The model under review builds one solid part; all positions refer to its coordinate system, in mm. A direction names the side the tool comes from. Round coordinates to 2 decimals unless told otherwise and drop trailing zeros. Write each loop counter-clockwise with the first axis right and the second up, starting at its lowest first coordinate (ties: lowest second). Pieces come first, ordered by that corner, then holes. Notation, with made-up numbers: (47, 83) -> (72, 83) arc R31 cw to (72, 120) -> close; hole circle Ø11 at (63.25, 89). An arc over 180 degrees is marked (long way). Answer in a Markdown table with one row per item. Add a question column.
```python
from build123d import *

# Parameters (mm, degrees)
BASE_FLANGE1_DEPTH = 70
CUT_EXTRUDE1_REACH = 78.974
CUT_EXTRUDE2_REACH = 78.348
SKETCH7_R          = 9
CUT_EXTRUDE3_REACH = 75.866
SKETCH8_R          = 3.25
FILLET1_R          = 1


# Sheet-metal steps are written as plain solids
with BuildPart() as part:
    # Sketch1 → Base-Flange1 (new body)
    with BuildSketch(Plane(origin=(0, 0, 0), x_dir=(0, 0, -1), z_dir=(1, 0, 0))):
        with BuildLine():
            Line((-12.5, 20), (-12.5, 3))
            ThreePointArc((-12.5, 3), (-11.621320344, 0.878679656), (-9.5, 0))
            Line((-9.5, 0), (9.5, 0))
            ThreePointArc((9.5, 0), (11.621320344, 0.878679656), (12.5, 3))
            Line((12.5, 3), (12.5, 20))
            Line((12.5, 20), (10.5, 20))
            Line((10.5, 20), (10.5, 3))
            ThreePointArc((10.5, 3), (10.207106781, 2.292893219), (9.5, 2))
            Line((9.5, 2), (-9.5, 2))
            ThreePointArc((-9.5, 2), (-10.207106781, 2.292893219), (-10.5, 3))
            Line((-10.5, 3), (-10.5, 20))
            Line((-10.5, 20), (-12.5, 20))
        make_face()
    extrude(amount=BASE_FLANGE1_DEPTH)

    # Sketch6 → Cut-Extrude1 (cut, up to next)
    with BuildSketch(Plane.XY.offset(12.5), mode=Mode.PRIVATE) as cut_extrude1_sk1:
        Polygon((35, 8.952994616), (45, 14.726497308), (45, 26.273502692), (35, 32.047005384), (25, 26.273502692), (25, 14.726497308), align=None)
    cut_extrude1_tool1 = extrude(cut_extrude1_sk1.sketch, amount=-CUT_EXTRUDE1_REACH, mode=Mode.PRIVATE) & part.part
    add(cut_extrude1_tool1.solids().sort_by_distance((35, 20.5, 12.5))[0], mode=Mode.SUBTRACT)

    # Sketch7 → Cut-Extrude2 (cut, up to next)
    with BuildSketch(Plane.XY.offset(-10.5), mode=Mode.PRIVATE) as cut_extrude2_sk1:
        with Locations((35, 20.5)):
            Circle(SKETCH7_R)
    cut_extrude2_tool1 = extrude(cut_extrude2_sk1.sketch, amount=-CUT_EXTRUDE2_REACH, mode=Mode.PRIVATE) & part.part
    add(cut_extrude2_tool1.solids().sort_by_distance((35, 20.5, -10.5))[0], mode=Mode.SUBTRACT)

    # Sketch8 → Cut-Extrude3 (cut, up to next)
    with BuildSketch(Plane.XZ, mode=Mode.PRIVATE) as cut_extrude3_sk1:
        with Locations(Location((65, 0, 0), (0, 0, 270))):
            Circle(SKETCH8_R)
    cut_extrude3_tool1 = extrude(cut_extrude3_sk1.sketch, amount=-CUT_EXTRUDE3_REACH, mode=Mode.PRIVATE) & part.part
    # Sketch8 → Cut-Extrude3 (cut, up to next)
    with BuildSketch(Plane.XZ, mode=Mode.PRIVATE) as cut_extrude3_sk2:
        with Locations(Location((5, 0, 0), (0, 0, 270))):
            Circle(SKETCH8_R)
    cut_extrude3_tool2 = extrude(cut_extrude3_sk2.sketch, amount=-CUT_EXTRUDE3_REACH, mode=Mode.PRIVATE) & part.part
    add(cut_extrude3_tool1.solids().sort_by_distance((65, 0, 0))[0], mode=Mode.SUBTRACT)
    add(cut_extrude3_tool2.solids().sort_by_distance((5, 0, 0))[0], mode=Mode.SUBTRACT)

    # Fillet1
    fillet1_edges = [part.edges().sort_by_distance(p)[0] for p in [
        (0, 20, -11.5),
        (0, 20, 11.5),
        (70, 20, -11.5),
        (70, 20, 11.5),
    ]]
    fillet(fillet1_edges, radius=FILLET1_R)


solid = part.part
```
1. Mouldability with a two-part tool opening along X and no side actions: class faces 1 (the flat face through (70, 1.8, -0.9)), 2 (the flat face through (39.93, 11.8, 11.51)), 3 (the flat face through (35, 0, 0)) as pulls with the +X half, pulls with the -X half, needs draft (parallel to the pull), parting line crosses it, or undercut.
2. Add section A-A on x = 65. Write out the cut boundary in (y, z).
3. Add section C-C on x = 57.5. Write out the cut boundary in (y, z), plus the area to 3 significant figures.
4. Add section D-D on y = 6. Write out the cut boundary in (x, z).
5. For L1, parallel to X at y = 0.7, z = 0; L2, parallel to Z at x = 45.5, y = 3.25; L3, parallel to X at y = 17.25, z = 11.5, list the stretches that pass through material, from the lowest coordinate up.
6. Insertion check: pin 1 Ø6 at (x, z) = (57, 6.5) entering from +Y. The pin has a flat end and moves straight along its axis. Give the tip position at first contact, or say it passes through.
7. Tool access review of faces 4 (the cylindrical face through (34.51, 0.9, 11.64)), 5 (the flat face through (35, 8, 10.5)), 6 (the flat face through (29.93, 11.88, 11.51)): name each direction out of +Z, -Z, +X, -X, +Y, -Y from which nothing blocks a thin tool from reaching the whole face with its end or side.
8. Add section B-B on y = 10. Write out the cut boundary in (x, z), plus the area to 3 significant figures.
Filled in:
| question | item | result |
|---|---|---|
| 1 | face 1 | pulls with the +X half |
| 1 | face 2 | undercut |
| 1 | face 3 | needs draft |
| 2 | outline | (0, -9.5) arc R3 ccw to (3, -12.5) -> (20, -12.5) -> (20, -10.5) -> (3, -10.5) arc R1 cw to (2, -9.5) -> (2, -3.25) -> (0, -3.25) -> close; (0, 3.25) -> (2, 3.25) -> (2, 9.5) arc R1 cw to (3, 10.5) -> (20, 10.5) -> (20, 12.5) -> (3, 12.5) arc R3 ccw to (0, 9.5) -> close |
| 3 | outline | (0, -9.5) arc R3 ccw to (3, -12.5) -> (20, -12.5) -> (20, -10.5) -> (3, -10.5) arc R1 cw to (2, -9.5) -> (2, 9.5) arc R1 cw to (3, 10.5) -> (20, 10.5) -> (20, 12.5) -> (3, 12.5) arc R3 ccw to (0, 9.5) -> close |
| 3 | area | 119 mm² |
| 4 | outline | (0, -12.5) -> (70, -12.5) -> (70, -10.5) -> (0, -10.5) -> close; (0, 10.5) -> (70, 10.5) -> (70, 12.5) -> (0, 12.5) -> close |
| 5 | L1 | 0 to 1.75, 8.25 to 61.75, 68.25 to 70 |
| 5 | L2 | -12.5 to -10.5, 10.5 to 12.5 |
| 5 | L3 | 0 to 25, 45 to 70 |
| 6 | pin 1 | y = 2 |
| 7 | face 4 | +Z, +X, -X, -Y |
| 7 | face 5 | +X, -X, +Y |
| 7 | face 6 | +Z, +Y |
| 8 | outline | (0, -12.5) -> (70, -12.5) -> (70, -10.5) -> (0, -10.5) -> close; (0, 10.5) -> (33.19, 10.5) -> (33.19, 12.5) -> (0, 12.5) -> close; (36.81, 10.5) -> (70, 10.5) -> (70, 12.5) -> (36.81, 12.5) -> close |
| 8 | area | 273 mm² |
